The model under review builds one solid part; all positions refer to its coordinate system, in mm. Round coordinates to 2 decimals unless told otherwise and drop trailing zeros. Write each loop counter-clockwise with the first axis right and the second up, starting at its lowest first coordinate (ties: lowest second). Pieces come first, ordered by that corner, then holes. Notation, with made-up numbers: M -23.5,-29.5 L 7.5,-29.5 A22 cw 7.5,-15.5 Z; hole C -14.5,64.25 d3. An arc over 180 degrees is marked long. One line per item, written item: value. Start each with the question number.
1) Wall thickness on probe 1 along X at (y, z) = (205, 703.5); probe 2 along Y at (x, z) = (136, 876); probe 3 along X at (y, z) = (228.5, 668): over which ranges is each line inside the solid? List them lowest first.
2) Take a section at D-D, the plane z = 830. Write out the cut boundary in (x, y), and give its area (3 significant figures).
3) Take a section at B-B, the plane x = -83. Write out the cut boundary in (y, z).
4) Take a section at A-A, the plane z = 657. Write out the cut boundary in (x, y).
5) For P1, Ø3, axis at x = -121, y = 113, coming from the +Z side; P2, Ø3, axis at y = -84.5, z = 778, coming from the -X side; P3, Ø2, axis at x = -48.5, z = 752.5, coming from the +Y side, all flat-tipped, find the tip position at first contact; note any pin that passes through.
6) Take a section at C-C, the plane y = -290. Write out the cut boundary in (x, z).
from build123d import *

# Parameters (mm, degrees)
F3_DEPTH = 1100
F5_DEPTH = 1100
F6_R     = 1000
F7_DEPTH = 577.3502691896


with BuildPart() as f1:
    # F0 (on Front) → F1 (revolve)
    with BuildSketch(Plane.XZ):
        with BuildLine():
            Line((0, -1000), (0, 1000))
            ThreePointArc((0, 1000), (-1000, 0), (0, -1000))
        make_face()
    revolve(axis=Axis((0, 0, 0), (0, 0, -1)))

    # F2 (on Front) → F3 (cut, symmetric)
    with BuildSketch(Plane.XZ):
        Polygon((0, 0), (-1100, 1100), (-1100, -1100), (1100, -1100), (1100, 1100), align=None)
    extrude(amount=F3_DEPTH, both=True, mode=Mode.SUBTRACT)

    # F4 (on Right) → F5 (cut, symmetric)
    with BuildSketch(Plane.YZ):
        Polygon((0, 0), (-1100, 1100), (-1100, -1100), (1100, -1100), (1100, 1100), align=None)
    extrude(amount=F5_DEPTH, both=True, mode=Mode.SUBTRACT)

    # F6 (on Top) → F7 (cut, through all)
    with BuildSketch(Plane.XY):
        Circle(F6_R)
    extrude(amount=F7_DEPTH, mode=Mode.SUBTRACT)


solid = f1.part
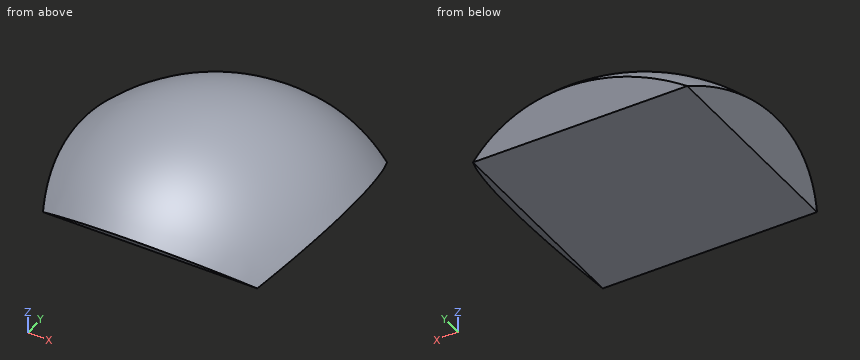
Checked values:
1. probe 1: x = -680.49 to 680.49
1. probe 2: y = -462.74 to 462.74
1. probe 3: x = -668 to 668
2. outline: C 0,0 d1115.53
2. area: 977,000 mm2
3. outline: M -704.67,704.67 L -577.35,577.35 L 577.35,577.35 L 704.67,704.67 A996.55 ccw Z
4. outline: M -657,-369.73 A753.89 ccw -369.73,-657 L 369.73,-657 A753.89 ccw 657,-369.73 L 657,369.73 A753.89 ccw 369.73,657 L -369.73,657 A753.89 ccw -657,369.73 Z
5. P1: stops at z = 986.45
5. P2: stops at x = -624.44
5. P3: stops at y = 657.95
6. outline: M -676.72,676.72 L -577.35,577.35 L 577.35,577.35 L 676.72,676.72 A957.03 ccw Z
